Here's how the part is built. I have some questions about the finished solid (model axes, mm). A direction names the side the tool comes from. Round coordinates to 2 decimals unless told otherwise and drop trailing zeros. Answer in a Markdown table with one row per item.
from build123d import *

# Parameters (mm, degrees)
REVOLVE5_ANGLE        = 90
SKETCH1_24_ONE_SIDE_W = 2.54
SKETCH1_24_ONE_SIDE_H = 28.448


with BuildPart() as part:
    # Sketch1 → Revolve4 (revolve)
    with BuildSketch(Plane.XY):
        Polygon((9.525, 101.6), (9.525, 104.902), (2.54, 104.902), (0, 104.902), (0, 101.6), (6.35, 101.6), align=None)
    revolve(axis=Axis((0, 133.35, 0), (0, -1, 0)))

    # Sketch1_21 → Revolve5 (revolve, symmetric)
    with BuildSketch(Plane.XY) as revolve5_sk:
        Polygon((9.525, 95.25), (9.525, 101.6), (6.35, 101.6), (6.35, 97.79), (3.937, 97.79), (3.937, 97.536), (3.937, 95.504), (3.937, 95.25), align=None)
        Polygon((-6.35, 97.79), (-6.35, 101.6), (-9.525, 101.6), (-9.525, 95.25), (-3.937, 95.25), (-3.937, 95.504), (-3.937, 97.536), (-3.937, 97.79), align=None)
    revolve(axis=Axis((0, 133.35, 0), (0, -1, 0)), revolution_arc=REVOLVE5_ANGLE / 2)
    revolve(revolve5_sk.sketch, axis=Axis((0, 133.35, 0), (0, 1, 0)), revolution_arc=REVOLVE5_ANGLE / 2)

    # Sketch1_24 one side → Revolve7 (revolve)
    with BuildSketch(Plane.XY):
        with Locations((1.27, 119.126)):
            Rectangle(SKETCH1_24_ONE_SIDE_W, SKETCH1_24_ONE_SIDE_H)
    revolve(axis=Axis((0, 133.35, 0), (0, -1, 0)))

    # Sketch1_32 one side → Revolve8 (revolve)
    with BuildSketch(Plane.XY):
        with BuildLine():
            ThreePointArc((7.619929338, 133.38281581), (5.07970677, 133.406330996), (2.54, 133.35))
            Line((2.54, 133.35), (2.54, 130.866278235))
            Line((2.54, 130.866278235), (5.08, 130.866278235))
            ThreePointArc((5.08, 130.866278235), (6.350063158, 130.864440752), (7.619929338, 130.841997813))
            Line((7.619929338, 130.841997813), (7.619929338, 133.38281581))
        make_face()
    revolve(axis=Axis((0, 133.35, 0), (0, -1, 0)))

    # Sketch1_36 → Revolve9 (revolve)
    with BuildSketch(Plane.XY):
        with BuildLine():
            Line((7.619929338, 133.38281581), (7.619929338, 130.841997813))
            ThreePointArc((7.619929338, 130.841997813), (44.514359536, 120.511244071), (72.087103792, 93.909228608))
            Line((72.087103792, 93.909228608), (74.244401193, 95.25))
            ThreePointArc((74.244401193, 95.25), (45.748561471, 122.731465818), (7.619929338, 133.38281581))
        make_face()
    revolve(axis=Axis((0, 133.35, 0), (0, -1, 0)))


solid = part.part
1) I need wall thicknesses on line 1 (X direction, y = 103.5, z = 5); line 2 (X direction, y = 103, z = 45); line 3 (Z direction, x = -27, y = 106). Which ranges of each line are inside material? Lowest first, please. Write a range as [from, to].
Response:
| item | result |
|---|---|
| line 1 | x = [-68.19, -64.87], [-8.11, 8.11], [64.87, 68.19] |
| line 2 | x = [-52.01, -47.58], [47.58, 52.01] |
| line 3 | z = [-60.51, -56.73], [56.73, 60.51] |
2) For pin 1 (4 mm diameter, centred on x = -0.5, z = 0.5, fed in from +Y); pin 2 (5 mm diameter, centred on x = -0.5, z = -2, fed in from -Y); pin 3 (12 mm diameter, centred on x = 24, z = 11.5, fed in from -Y), each with a flat end and sliding along its axis, tell me the tip position at first contact or that it passes through.
Response:
| item | result |
|---|---|
| pin 1 | stops at y = 133.36 |
| pin 2 | stops at y = 95.25 |
| pin 3 | stops at y = 126.06 |
3) I want a section at A-A, the plane y = 126. Count the separate pieces of the cut face and the enclosed holes in it, and give its area (3 significant figures).
Response:
| item | result |
|---|---|
| separate pieces | 2 |
| enclosed holes | 1 |
| area | 1,520 mm^2 |
4) We'd pull the mould along X, two halves only. Please class faces 1 (the face through (-15.66, 93.99, -70.5)), 2 (the face through (-0.33, 118.07, 2.52)): +X half, -X half, draft (parallel to the pull), parting line (faces both ways), or undercut.
Response:
| item | result |
|---|---|
| face 1 | parting line |
| face 2 | undercut |
5) Which directions (+Z, -Z, +X, -X, +Y, -Y) give clear straight access to the entire face, cutting with the end or side of a thin tool? Please do faces 3 (the face through (5, 97.79, 0)), 4 (the face through (-6, 95.25, 0)).
Response:
| item | result |
|---|---|
| face 3 | none |
| face 4 | -Y |
